Read the model definition and answer for the solid it produces. Units are mm, in the model's axes. A direction names the side the tool comes from. Coordinates: 2 decimals unless noted, no trailing zeros. Loops run counter-clockwise (first coordinate to the right, second up) from the corner with the lowest first, then second, coordinate; pieces in that order, holes last. Notation, with made-up numbers: (29.25, -6) -> (69.25, -6) arc R20 ccw to (69.25, 26) -> close; hole circle Ø6 at (-1.75, -39). An arc over 180 degrees is marked (long way). Answer as a JSON object with one key per item and string values. Group by question number.
Q1. The part is cut by section A-A on z = -18. Write down the section's boundary in (x, y), and give its area (3 significant figures).
Q2. Straight lines are drawn through the part: line 1 along X through (y, z) = (38.5, -24); line 2 along X through (y, z) = (-1.75, -18); line 3 along Z through (x, y) = (-20, 54). For each, find the intervals that lie inside material, in ascending order. Write a range as [from, to].
Q3. Each of these flat-tipped pins is pushed along its axis until it touches: P1, Ø6, axis at x = -12, z = -5, coming from the +Y side; P2, Ø1.5, axis at x = -23.5, z = 4.5, coming from the -Y side; P3, Ø5.5, axis at x = -10, y = 27, coming from the +Z side. Where does it stop, or does it pass through?
Q4. Determine the mould class of faces 5 (the flat face through (-21, 11, -10)), 6 (the flat face through (-9, 16, -27)), 7 (the flat face through (-27, 52, -2)) for opening direction X: released by +X, released by -X, zero draft, split by the parting line, or undercut.
Q5. The part is cut by section C-C on y = 22.5. Write down the section's boundary in (x, z), and give its area (3 significant figures).
Q6. For faces 1 (the flat face through (-9, 16, 0)), 2 (the flat face through (-1.3, 14.04, -13.56)), 3 (the flat face through (-24.16, 26.84, -6.9)), 4 (the flat face through (-9, 0.5, -18)), determine the directions among +Z, -Z, +X, -X, +Y, -Y from which every point of the face is accessible in a straight line to the end or side of a thin tool.
Q7. The part is cut by section B-B on x = -3. State how many separate pieces and enclosed holes the cut face has, and give its area (3 significant figures).
from build123d import *

# Parameters (mm, degrees)
BOSS_EXTRUDE1_DEPTH     = 30
SKETCH6_R               = 7.75
CUT_EXTRUDE3_DEPTH      = 0.5
BOSS_EXTRUDE2_DEPTH     = 15
BOSS_EXTRUDE3_DEPTH     = 15
CHAMFER1_SIZE           = 5
CHAMFER1_SIZE2          = 10.251519208
BOSS_EXTRUDE5_DEPTH     = 15
BOSS_EXTRUDE6_REACH     = 75.607
SKETCH10_R              = 3.5
BOSS_EXTRUDE7_REACH     = 62.698
SKETCH18_W              = 10
SKETCH18_H              = 10.251519208
CUT_EXTRUDE4_DEPTH      = 74.607064878
CUT_EXTRUDE4_DEPTH_BACK = 74.607064878
FILLET4_R               = 7
FILLET5_R               = 7
FILLET6_R               = 7
FILLET7_R               = 7
BOSS_EXTRUDE8_REACH     = 75.607
FILLET9_R               = 7
CUT_EXTRUDE5_DEPTH      = 23
FILLET12_R              = 7
BOSS_EXTRUDE9_REACH     = 75.607
BOSS_EXTRUDE10_START    = 10
SKETCH24_R              = 7.75
BOSS_EXTRUDE10_DEPTH    = 10
SKETCH25_W              = 18.768324379
SKETCH25_H              = 6
CUT_EXTRUDE6_DEPTH      = 10
SKETCH26_W              = 18.768324379
SKETCH26_H              = 6
CUT_EXTRUDE7_DEPTH      = 10


with BuildPart() as part:
    # Sketch1 → Boss-Extrude1 (new body)
    with BuildSketch(Plane(origin=(0, 0, 0), x_dir=(1, 0, 0), z_dir=(0, 1, 0))):
        Polygon((-30.5, 27), (12.5, 27), (12.5, 14), (0, 0), (-18, 0), (-30.5, 14), align=None)
    extrude(amount=BOSS_EXTRUDE1_DEPTH)

    # Sketch6 → Cut-Extrude3 (cut)
    with BuildSketch(Plane.XZ):
        with Locations(Location((-9, -18, 0), (0, 0, 270))):
            Circle(SKETCH6_R)
    extrude(amount=-CUT_EXTRUDE3_DEPTH, mode=Mode.SUBTRACT)

    # Sketch7 → Boss-Extrude2 (add)
    with BuildSketch(Plane(origin=(0, 30, 0), x_dir=(1, 0, 0), z_dir=(0, 1, 0))):
        Polygon((-30.5, 27), (-30.5, 14), (-18, 0), (0, 0), (12.5, 14), (12.5, 27), align=None)
    extrude(amount=BOSS_EXTRUDE2_DEPTH)

    # Sketch8 → Boss-Extrude3 (add)
    with BuildSketch(Plane(origin=(0, 45, 0), x_dir=(1, 0, 0), z_dir=(0, 1, 0))):
        Polygon((-30.5, 27), (-30.5, 9), (-23.5, -5), (-20.5, -5), (-20.5, 27), align=None)
    extrude(amount=BOSS_EXTRUDE3_DEPTH)

    # Chamfer1
    chamfer1_edges = [part.edges().sort_by_distance(p)[0] for p in [
        (-4, 45, -27),
    ]]
    chamfer1_side = [part.faces().sort_by_distance(p)[0] for p in [
        (-10.18705036, 24.658273381, -27),
    ]]
    chamfer(chamfer1_edges, length=CHAMFER1_SIZE, length2=CHAMFER1_SIZE2, reference=chamfer1_side[0])

    # Sketch12 → Boss-Extrude5 (add)
    with BuildSketch(Plane(origin=(0, 45, 0), x_dir=(1, 0, 0), z_dir=(0, 1, 0))):
        Polygon((12.5, 9), (12.5, 27), (2.5, 27), (2.5, -5), (5.5, -5), align=None)
    extrude(amount=BOSS_EXTRUDE5_DEPTH)

    # Sketch10 → Boss-Extrude6 (add, up to next)
    with BuildSketch(Plane(origin=(-20.5, 0, 0), x_dir=(0, 0, -1), z_dir=(1, 0, 0)), mode=Mode.PRIVATE) as boss_extrude6_sk1:
        with Locations(Location((1.594739548, 53.968499846, 0), (0, 0, 180))):
            Circle(SKETCH10_R)
    boss_extrude6_tool1 = extrude(boss_extrude6_sk1.sketch, amount=BOSS_EXTRUDE6_REACH, mode=Mode.PRIVATE) - part.part
    add(boss_extrude6_tool1.solids().sort_by_distance((-20.5, 53.9685, -1.59474))[0])

    # Boss-Extrude7: up to this face of the body (flat: up to its plane)
    boss_extrude7_end = Plane(part.part.faces().sort_by_distance((-4, 42.5, -21.874240396))[0])
    # Sketch18 → Boss-Extrude7 (add, up to the picked face)
    with BuildSketch(Plane.XZ.offset(-45), mode=Mode.PRIVATE) as boss_extrude7_sk1:
        with Locations((7.5, -21.874240396)):
            Rectangle(SKETCH18_W, SKETCH18_H)
    boss_extrude7_tool1 = split(extrude(boss_extrude7_sk1.sketch, amount=BOSS_EXTRUDE7_REACH, mode=Mode.PRIVATE), bisect_by=boss_extrude7_end, keep=Keep.BOTH, mode=Mode.PRIVATE)
    add(boss_extrude7_tool1.solids().sort_by(Axis((7.5, 45, -21.87424), (0, -1, 0)))[0])

    # Sketch19 → Cut-Extrude4 (cut, two sides: drawn at the far end of the back side and taken through both)
    with BuildSketch(Plane(origin=(-20.5, 0, 0), x_dir=(0, 0, -1), z_dir=(1, 0, 0)).offset(-CUT_EXTRUDE4_DEPTH_BACK)):
        Polygon((1.052419117, 60), (27, 47.344519209), (30.679345013, 60.875953777), (1.052419117, 61.751907555), align=None)
    extrude(amount=CUT_EXTRUDE4_DEPTH + CUT_EXTRUDE4_DEPTH_BACK, mode=Mode.SUBTRACT)

    # Fillet4
    # the kernel refuses this fillet: 7 mm, written as the material it takes off along each edge
    with BuildSketch(Plane(origin=(-40.838917655, 60, 5), x_dir=(0, 0, -1), z_dir=(1, 0, 0))) as fillet4_piece_1:
        with BuildLine():
            CenterArc((7, -6.935567062), FILLET4_R, 97.779940417, 82.220059583)
            Line((0, -6.935567062), (-0.14, -6.935567062))
            Line((-0.14, -6.935567062), (-0.14, 0))
            Line((-0.14, 0), (0, 0.14))
            ThreePointArc((0, 0.14), (3.026209558, 0.14), (6.033467499, 0.138711341))
            Line((6.033467499, 0.138711341), (6.052419117, 0))
        make_face()
    extrude(amount=37.677835309, mode=Mode.SUBTRACT)

    # Fillet5
    # the kernel refuses this fillet: 7 mm, written as the material it takes off along each edge
    with BuildSketch(Plane(origin=(-14.838917655, 60, 5), x_dir=(0, 0, -1), z_dir=(1, 0, 0))) as fillet5_piece_1:
        with BuildLine():
            CenterArc((7, -6.935567062), FILLET5_R, 97.779940417, 82.220059583)
            Line((0, -6.935567062), (-0.14, -6.935567062))
            Line((-0.14, -6.935567062), (-0.14, 0))
            Line((-0.14, 0), (0, 0.14))
            ThreePointArc((0, 0.14), (3.026209558, 0.14), (6.033467499, 0.138711341))
            Line((6.033467499, 0.138711341), (6.052419117, 0))
        make_face()
    extrude(amount=37.677835309, mode=Mode.SUBTRACT)

    # Fillet6
    # the kernel refuses this fillet: 7 mm, written as the material it adds along each edge
    with BuildSketch(Plane(origin=(-9.155275963, 45, 10.253909078), x_dir=(0, -1, 0), z_dir=(0.6660157693088524, 0, -0.7459376616259147))) as fillet6_piece_1_section:
        with BuildLine():
            CenterArc((FILLET6_R, -FILLET6_R), FILLET6_R, 90, 90)
            Line((0, -FILLET6_R), (0, 0))
            Line((0, 0), (FILLET6_R, 0))
        make_face()
    fillet6_piece_1 = extrude(amount=50.014659503, mode=Mode.PRIVATE)
    fillet6_piece_1 = split(fillet6_piece_1, bisect_by=Plane(origin=(12.5, 45, 10.253909078), z_dir=(-1, 0, 0)), keep=Keep.TOP, mode=Mode.PRIVATE)
    fillet6_piece_1 = split(fillet6_piece_1, bisect_by=Plane(origin=(2.5, 45, 10.253909078), z_dir=(1, 0, 0)), keep=Keep.TOP, mode=Mode.PRIVATE)
    fillet6_piece_1 = split(fillet6_piece_1, bisect_by=Plane(origin=(0.467381176, 45, 15.065237648), z_dir=(-0.8944271909999162, 0, -0.4472135954999575)), keep=Keep.TOP, mode=Mode.PRIVATE)
    fillet6_piece_1 = split(fillet6_piece_1, bisect_by=Plane(origin=(-9.155275963, 45, 5), z_dir=(0, 0, -1)), keep=Keep.TOP, mode=Mode.PRIVATE)
    add(fillet6_piece_1)

    # Fillet7
    # the kernel refuses this fillet: 7 mm, written as the material it adds along each edge
    with BuildSketch(Plane(origin=(-42.155275963, 45, -27.053909078), x_dir=(-0.7459376616259148, 0, 0.6660157693088522), z_dir=(0.6660157693088522, 0, 0.7459376616259148))) as fillet7_piece_1_section:
        with BuildLine():
            CenterArc((FILLET7_R, FILLET7_R), FILLET7_R, 180, 90)
            Line((0, FILLET7_R), (0, 0))
            Line((0, 0), (FILLET7_R, 0))
        make_face()
    fillet7_piece_1 = extrude(amount=50.014659503, mode=Mode.PRIVATE)
    fillet7_piece_1 = split(fillet7_piece_1, bisect_by=Plane(origin=(-30.5, 45, -27.053909078), z_dir=(1, 0, 0)), keep=Keep.TOP, mode=Mode.PRIVATE)
    fillet7_piece_1 = split(fillet7_piece_1, bisect_by=Plane(origin=(-42.155275963, 45, 5), z_dir=(0, 0, -1)), keep=Keep.TOP, mode=Mode.PRIVATE)
    fillet7_piece_1 = split(fillet7_piece_1, bisect_by=Plane(origin=(-40.052618824, 45, -28.105237648), z_dir=(0.8944271909999161, 0, -0.4472135954999577)), keep=Keep.TOP, mode=Mode.PRIVATE)
    fillet7_piece_1 = split(fillet7_piece_1, bisect_by=Plane(origin=(-20.5, 45, -27.053909078), z_dir=(-1, 0, 0)), keep=Keep.TOP, mode=Mode.PRIVATE)
    add(fillet7_piece_1)

    # Sketch21 → Boss-Extrude8 (add, up to next)
    with BuildSketch(Plane(origin=(-20.5, 0, 0), x_dir=(0, 0, -1), z_dir=(1, 0, 0)), mode=Mode.PRIVATE) as boss_extrude8_sk1:
        with BuildLine():
            Line((2.8, 45), (-5, 45))
            Line((-5, 45), (-5, 44.763260828))
            add(Edge.make_bspline(
                [(2.8, 38), (2.8, 43.376764541), (-5, 44.763260828)],
                knots=[0, 0, 0, 1.309981256, 1.309981256, 1.309981256], degree=2, weights=[1, 0.793053637, 1]))
            Line((2.8, 38), (2.8, 45))
        make_face()
    boss_extrude8_tool1 = extrude(boss_extrude8_sk1.sketch, amount=BOSS_EXTRUDE8_REACH, mode=Mode.PRIVATE) - part.part
    add(boss_extrude8_tool1.solids().sort_by_distance((-20.5, 43.416068, -0.535904))[0])

    # Fillet9
    fillet9_edges = [part.edges().sort_by_distance(p)[0] for p in [
        (-25.5, 47.344519209, -27),
        (7.5, 47.344519209, -27),
        (-9, 40, -27),
    ]]
    fillet(fillet9_edges, radius=FILLET9_R)

    # Sketch22 → Cut-Extrude5 (cut)
    with BuildSketch(Plane.ZY.offset(-2.5)):
        Polygon((5, 51.374505428), (-27, 35.767062594), (-27, 42.970433745), (-2.018410751, 49.666818357), align=None)
    extrude(amount=CUT_EXTRUDE5_DEPTH, mode=Mode.SUBTRACT)

    # Fillet12
    # the kernel refuses this fillet: 7 mm, written as the material it takes off along each edge
    with BuildSketch(Plane(origin=(2.5, 35.767763648, -26.998562626), x_dir=(0, -0.9999999460246048, -0.0003285586515390651), z_dir=(-1, 0, 0))) as fillet12_piece_1:
        with BuildLine():
            CenterArc((4.372486843, 6.999999622), FILLET12_R, 206.018825024, 64)
            Line((-1.918062927, 3.929334614), (-2.547117904, 3.622268114))
            Line((-2.547117904, 3.622268114), (-0.629054977, -0.307066501))
            Line((-0.629054977, -0.307066501), (-0.013954967, -0.699860885))
            ThreePointArc((-0.013954967, -0.699860885), (0.142079567, -0.70139073), (4.375016745, -0.699999962))
            Line((4.375016745, -0.699999962), (4.374786754, 0))
        make_face()
    extrude(amount=23, mode=Mode.SUBTRACT)
    with BuildSketch(Plane(origin=(2.5, 45, -8.069672968), x_dir=(0, -0.438371146789077, -0.8987940462991671), z_dir=(-1, 0, 0))) as fillet12_piece_2:
        with BuildLine():
            CenterArc((FILLET12_R * 0.230868191126, FILLET12_R), FILLET12_R, 244, 26)
            Line((-FILLET12_R * 0.207502955664, FILLET12_R * 0.101205953701), (0, 0))
            Line((0, 0), (FILLET12_R * 0.230868191126, 0))
        make_face()
    extrude(amount=23, mode=Mode.SUBTRACT)

    # Sketch23 → Boss-Extrude9 (add, up to next)
    with BuildSketch(Plane.ZY.offset(-2.5), mode=Mode.PRIVATE) as boss_extrude9_sk1:
        with BuildLine():
            Line((5, 45), (-1, 45))
            ThreePointArc((-1, 45), (2.755309717, 46.57305469), (5, 49.969849895))
            Line((5, 49.969849895), (5, 45))
        make_face()
    boss_extrude9_tool1 = extrude(boss_extrude9_sk1.sketch, amount=BOSS_EXTRUDE9_REACH, mode=Mode.PRIVATE) - part.part
    add(boss_extrude9_tool1.solids().sort_by_distance((2.5, 46.322933, 3.503714))[0])

    # Sketch24 → Boss-Extrude10 (add)
    with BuildSketch(Plane.XZ.offset(BOSS_EXTRUDE10_START)):
        Polygon((-30.5, -14), (-30.5, -27), (12.5, -27), (12.5, -14), (0, 0), (-18, 0), align=None)
        with Locations(Location((-9, -18, 0), (0, 0, 270))):
            Circle(SKETCH24_R, mode=Mode.SUBTRACT)
    extrude(amount=-BOSS_EXTRUDE10_DEPTH)

    # Sketch25 → Cut-Extrude6 (cut)
    with BuildSketch(Plane(origin=(0, 0, 0), x_dir=(0.6660157693088523, 0, -0.7459376616259148), z_dir=(0.7459376616259148, 0, 0.6660157693088523))):
        with Locations((9.38416219, 13.99928604)):
            Rectangle(SKETCH25_W, SKETCH25_H)
    extrude(amount=-CUT_EXTRUDE6_DEPTH, mode=Mode.SUBTRACT)

    # Sketch26 → Cut-Extrude7 (cut)
    with BuildSketch(Plane(origin=(-10.015613911, 0, 8.94251242), x_dir=(0.6660157693088522, 0, 0.7459376616259148), z_dir=(-0.7459376616259148, 0, 0.6660157693088522))):
        with Locations((-21.372446038, 14)):
            Rectangle(SKETCH26_W, SKETCH26_H)
    extrude(amount=-CUT_EXTRUDE7_DEPTH, mode=Mode.SUBTRACT)


solid = part.part
Final values:
{
 "1": {"outline": "(-30.5, -10) -> (-16.75, -10) -> (-16.75, 0.5) -> (-1.25, 0.5) -> (-1.25, -10) -> (12.5, -10) -> (12.5, 51.73) -> (2.5, 51.73) -> (2.5, 40.16) -> (-20.5, 40.16) -> (-20.5, 51.73) -> (-30.5, 51.73) -> close; hole (-26.02, 11) -> (-20.67, 11) -> (-20.67, 17) -> (-26.02, 17) -> close; hole (2.67, 11) -> (8.02, 11) -> (8.02, 17) -> (2.67, 17) -> close", "area": "2,160 mm2"},
 "2": {"line 1": "x = [-30.5, -20.5], [2.5, 12.5]", "line 2": "x = [-30.5, -16.75], [-1.25, 12.5]", "line 3": "z = [-5.09, 1.91]"},
 "3": {"P1": "stops at y = 57.44", "P2": "stops at y = 44.97", "P3": "stops at z = 0"},
 "4": {"face 5": "undercut", "face 6": "zero draft", "face 7": "released by -X"},
 "5": {"outline": "(-30.5, -27) -> (12.5, -27) -> (12.5, -14) -> (0, 0) -> (-18, 0) -> (-30.5, -14) -> close", "area": "986 mm2"},
 "6": {"face 1": "+Z, +X, -X, -Y", "face 2": "none", "face 3": "+Z, -X, -Y", "face 4": "-Y"},
 "7": {"separate pieces": "2", "enclosed holes": "1", "area": "1,290 mm2"}
}
